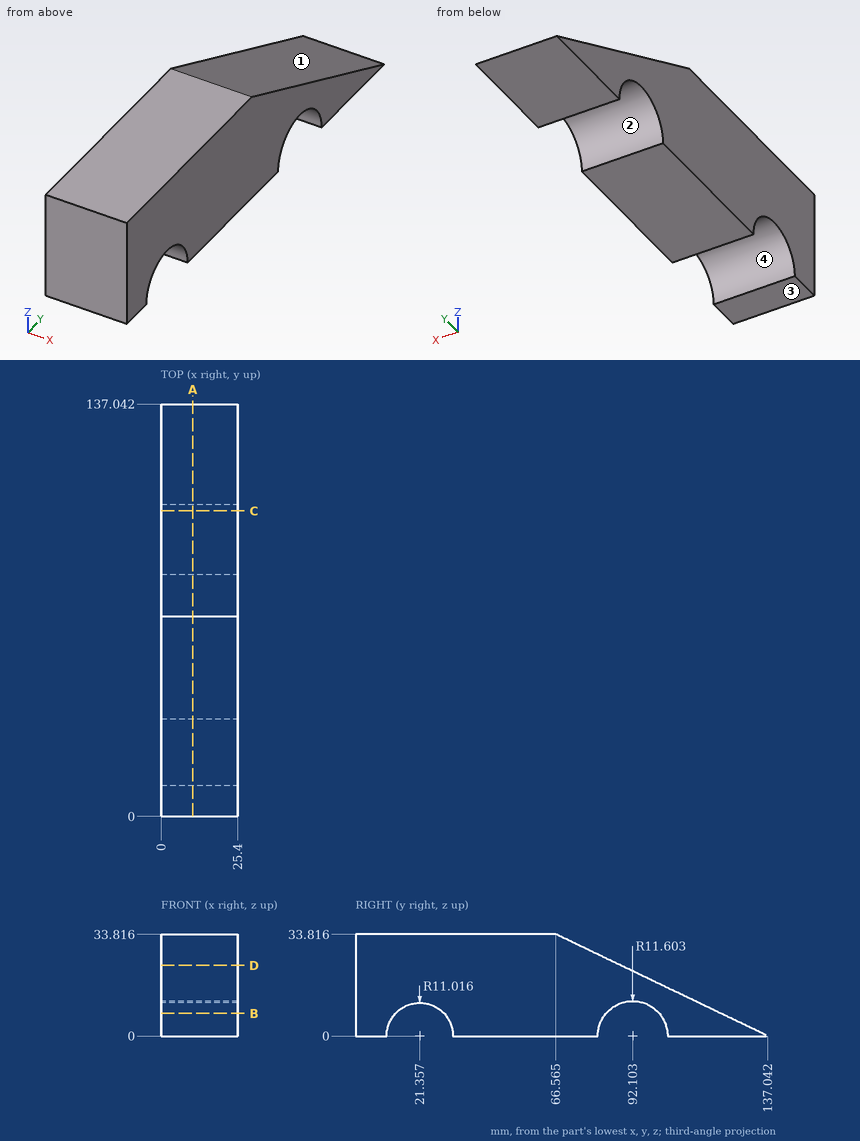
The drawing under review shows one solid part. Ordinate dimensions are in mm from its lowest x, y, z. Round coordinates to 2 decimals unless told otherwise and drop trailing zeros. Loops run counter-clockwise (first coordinate to the right, second up) from the corner with the lowest first, then second, coordinate; pieces in that order, holes last. Notation, with made-up numbers: (89, 37) -> (101, 37) arc R18 cw to (101, 71) -> close; hole circle Ø11 at (65.25, 11). An arc over 180 degrees is marked (long way). Answer in a Markdown table with one row per item.
1) For pin 1 Ø3 at (x, z) = (9, 3.5) entering from +Y (1 decimal); pin 2 Ø4 at (x, z) = (13.5, 27) entering from +Y (1 decimal); pin 3 Ø1 at (x, z) = (12.5, 16) entering from +Y (1 decimal), all flat-tipped, find the tip position at first contact; note any pin that passes through.
Taken from the geometry:
| item | result |
|---|---|
| pin 1 | stops at y = 132.9 |
| pin 2 | stops at y = 84.9 |
| pin 3 | stops at y = 104.7 |
2) Consider section D-D, the plane z = 23.5. Write out the cut boundary in (x, y) (1 decimal), plus the area to 3 significant figures.
Taken from the geometry:
| item | result |
|---|---|
| outline | (0, 0) -> (25.4, 0) -> (25.4, 88.1) -> (0, 88.1) -> close |
| area | 2,240 mm² |
3) Wall thickness on line 1 along Y through (x, z) = (8.75, 3) (1 decimal); line 2 along Y through (x, z) = (14.75, 8) (1 decimal); line 3 along Y through (x, z) = (22, 12) (1 decimal): over which ranges is each line inside the solid? List them lowest first.
Taken from the geometry:
| item | result |
|---|---|
| line 1 | y = 0 to 10.8, 32 to 80.9, 103.3 to 130.8 |
| line 2 | y = 0 to 13.8, 28.9 to 83.7, 100.5 to 120.4 |
| line 3 | y = 0 to 112 |
4) Consider section B-B, the plane z = 7.5. Count the separate pieces of the cut face and the enclosed holes in it, plus the area to 3 significant figures.
Taken from the geometry:
| item | result |
|---|---|
| separate pieces | 3 |
| enclosed holes | 0 |
| area | 2,220 mm² |
5) Draft analysis for pull direction Y (two halves, no side actions). For the marked faces 1, 2, 3 and 4, state which applies: pulls with the +Y half, pulls with the -Y half, needs draft (parallel to the pull), parting line crosses it, or undercut.
Taken from the geometry:
| item | result |
|---|---|
| face 1 | pulls with the +Y half |
| face 2 | undercut |
| face 3 | needs draft |
| face 4 | undercut |
6) Consider section C-C, the plane y = 101.5. Write out the cut boundary in (x, z) (1 decimal), plus the area to 3 significant figures.
Taken from the geometry:
| item | result |
|---|---|
| outline | (0, 6.8) -> (25.4, 6.8) -> (25.4, 17.1) -> (0, 17.1) -> close |
| area | 260 mm² |
7) Consider section A-A, the plane x = 10.5. Write out the cut boundary in (y, z) (1 decimal).
Taken from the geometry:
| item | result |
|---|---|
| outline | (0, 0) -> (10.3, 0) arc R11 cw to (32.4, 0) -> (80.5, 0) arc R11.6 cw to (103.7, 0) -> (137, 0) -> (66.6, 33.8) -> (0, 33.8) -> close |
